```python
from build123d import *

# Parameters (mm, degrees)
ESBO_O1_W                = 120
ESBO_O1_H                = 120
RESSALTO_EXTRUS_O1_DEPTH = 3
ESBO_O2_W                = 100
ESBO_O2_H                = 100
CORTE_EXTRUS_O1_DEPTH    = 4
ESBO_O3_R                = 1.5
CORTE_EXTRUS_O2_DEPTH    = 4
ESBO_O4_R                = 1.5
CORTE_EXTRUS_O3_DEPTH    = 4
ESBO_O5_R                = 1.5
CORTE_EXTRUS_O4_DEPTH    = 4
ESBO_O6_R                = 1.5
CORTE_EXTRUS_O5_DEPTH    = 4


with BuildPart() as part:
    # Esboço1 → Ressalto-extrusão1 (new body)
    with BuildSketch(Plane.XY):
        with Locations((53.473096186, -53.653846154)):
            Rectangle(ESBO_O1_W, ESBO_O1_H)
    extrude(amount=RESSALTO_EXTRUS_O1_DEPTH)

    # Esboço2 → Corte-extrusão1 (cut, through all)
    with BuildSketch(Plane.XY.offset(3)):
        with Locations((53.473096186, -53.653846154)):
            Rectangle(ESBO_O2_W, ESBO_O2_H)
    extrude(amount=-CORTE_EXTRUS_O1_DEPTH, mode=Mode.SUBTRACT)

    # Esboço3 → Corte-extrusão2 (cut, through all)
    with BuildSketch(Plane.XY.offset(3)):
        with Locations((-1.526903814, 1.346153846)):
            Circle(ESBO_O3_R)
        with Locations((-1.526903814, -108.653846154)):
            Circle(ESBO_O3_R)
        with Locations((-1.526903814, -33.653846154)):
            Circle(ESBO_O3_R)
        with Locations((-1.526903814, -53.653846154)):
            Circle(ESBO_O3_R)
        with Locations((-1.526903814, -73.653846154)):
            Circle(ESBO_O3_R)
        with Locations((108.473096186, -73.653846154)):
            Circle(ESBO_O3_R)
        with Locations((108.473096186, -53.653846154)):
            Circle(ESBO_O3_R)
        with Locations((108.473096186, -33.653846154)):
            Circle(ESBO_O3_R)
        with Locations((108.473096186, -108.653846154)):
            Circle(ESBO_O3_R)
        with Locations((108.473096186, 1.346153846)):
            Circle(ESBO_O3_R)
    extrude(amount=-CORTE_EXTRUS_O2_DEPTH, mode=Mode.SUBTRACT)

    # Esboço4 → Corte-extrusão3 (cut, through all)
    with BuildSketch(Plane.XY.offset(3)):
        with Locations((6.473096186, 1.346153846)):
            Circle(ESBO_O4_R)
    extrude(amount=-CORTE_EXTRUS_O3_DEPTH, mode=Mode.SUBTRACT)

    # Esboço5 → Corte-extrusão4 (cut, through all)
    with BuildSketch(Plane.XY.offset(3)):
        with Locations((73.473096186, -108.653846154)):
            Circle(ESBO_O5_R)
        with Locations((53.473096186, -108.653846154)):
            Circle(ESBO_O5_R)
        with Locations((33.473096186, -108.653846154)):
            Circle(ESBO_O5_R)
    extrude(amount=-CORTE_EXTRUS_O4_DEPTH, mode=Mode.SUBTRACT)

    # Esboço6 → Corte-extrusão5 (cut, through all)
    with BuildSketch(Plane.XY.offset(3)):
        with Locations((108.473096186, -23.653846154)):
            Circle(ESBO_O6_R)
        with Locations((108.473096186, -43.653846154)):
            Circle(ESBO_O6_R)
        with Locations((108.473096186, -63.653846154)):
            Circle(ESBO_O6_R)
        with Locations((108.473096186, -83.653846154)):
            Circle(ESBO_O6_R)
        with Locations((-1.526903814, -83.653846154)):
            Circle(ESBO_O6_R)
        with Locations((-1.526903814, -63.653846154)):
            Circle(ESBO_O6_R)
        with Locations((-1.526903814, -43.653846154)):
            Circle(ESBO_O6_R)
        with Locations((-1.526903814, -23.653846154)):
            Circle(ESBO_O6_R)
        with Locations((108.473096186, -8.653846154)):
            Circle(ESBO_O6_R)
        with Locations((108.473096186, -98.653846154)):
            Circle(ESBO_O6_R)
        with Locations((-1.526903814, -98.653846154)):
            Circle(ESBO_O6_R)
        with Locations((-1.526903814, -8.653846154)):
            Circle(ESBO_O6_R)
    extrude(amount=-CORTE_EXTRUS_O5_DEPTH, mode=Mode.SUBTRACT)


solid = part.part
```
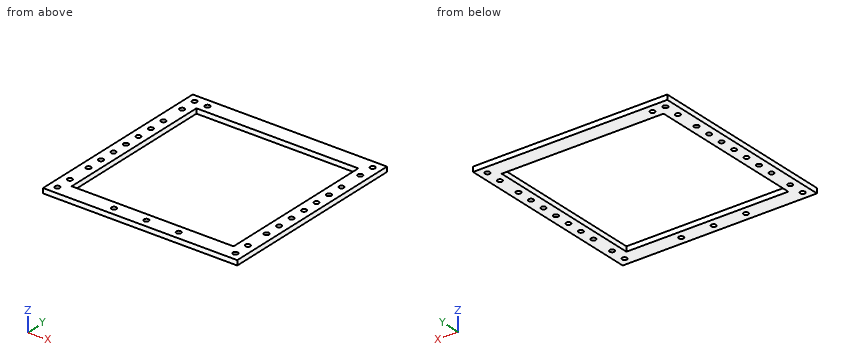
Design review of the part built by this model. Coordinates are the model's own, in mm. Give positions to 0.01 mm unless a question says otherwise; leave off trailing zeros. Loops run counter-clockwise (first coordinate to the right, second up) from the corner with the lowest first, then second, coordinate; pieces in that order, holes last. Notation, with made-up numbers: M -10.5,-3 L 2.5,-3 A29 cw 2.5,36 Z; hole C 45,85.5 d4. An arc over 180 degrees is marked long. Return JSON: item names as keys, results as strings. Group by question number.
Item 1: We need section C-C (z = 1.7). Give the number of separate pieces and of enclosed holes in the cut face, and give its area (3 significant figures).
Item 2: We need section B-B (x = 89). Give the boundary of the cut face in (y, z), and give its area (3 significant figures).
Item 3: We need section A-A (y = -48). Give the boundary of the cut face in (x, z).
Item 4: For probe 1 along X at (y, z) = (-79, 2.8); probe 2 along Y at (x, z) = (83.5, 1.8); probe 3 along X at (y, z) = (-83.5, 0.5), list the stretches that pass through material, from the lowest coordinate up.
Output:
{
 "1": {"separate pieces": "1", "enclosed holes": "27", "area": "4,220 mm^2"},
 "2": {"outline": "M -113.65,0 L -103.65,0 L -103.65,3 L -113.65,3 Z; M -3.65,0 L 6.35,0 L 6.35,3 L -3.65,3 Z", "area": "60.0 mm^2"},
 "3": {"outline": "M -6.53,0 L 3.47,0 L 3.47,3 L -6.53,3 Z; M 103.47,0 L 113.47,0 L 113.47,3 L 103.47,3 Z"},
 "4": {"probe 1": "x = -6.53 to 3.47, 103.47 to 113.47", "probe 2": "y = -113.65 to -103.65, -3.65 to 6.35", "probe 3": "x = -6.53 to -3.02, -0.03 to 3.47, 103.47 to 106.98, 109.97 to 113.47"}
}
